Study the drawing (mm; zero at the part's minimum x, y, z) and answer. Give positions to 0.01 mm unless a question says otherwise; leave off trailing zeros. Order: outer loops, then holes, each group sorted by start corner. A loop starts at its lowest first (then second) coordinate and runs counter-clockwise, first axis right, second up. Notation, with made-up numbers: (-19, -25.75) - (16, -25.75) arc R29 ccw to (16, -0.75) - close; hole circle Ø10 at (71, 51.25). An arc over 180 degrees is marked (long way). Put each result on its own line as item: value.
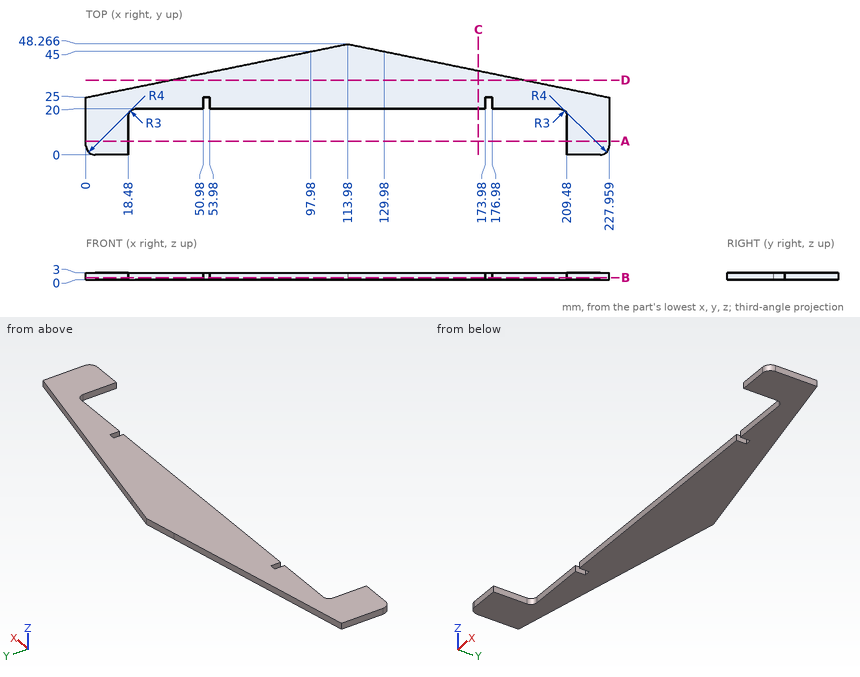
(1) Straight lines are drawn through the part: line 1 (X direction, y = 20.5, z = 1.2); line 2 (X direction, y = 13, z = 0.85); line 3 (Y direction, x = 138.5, z = 1). For each, find the intervals that lie inside material, in ascending order.
Geometry check:
line 1: x = 0 to 50.98, 53.98 to 173.98, 176.98 to 227.96
line 2: x = 0 to 18.48, 209.48 to 227.96
line 3: y = 20 to 43.26
(2) Section C-C, the plane x = 171 is taken. Write down the section's boundary in (y, z), then the cut area to 3 significant figures.
Geometry check:
outline: (20, 0) - (36.63, 0) - (36.63, 3) - (20, 3) - close
area: 49.9 mm²
(3) Section D-D, the plane y = 32.5 is taken. Write down the section's boundary in (x, z).
Geometry check:
outline: (36.74, 0) - (191.22, 0) - (191.22, 3) - (36.74, 3) - close
(4) Given pin 1 (1.5 mm diameter, centred on x = 117, z = 2, fed in from -Y); pin 2 (1.5 mm diameter, centred on x = 52, z = 1, fed in from -Y); pin 3 (3 mm diameter, centred on x = 182, y = 36.5, fed in from +Z), each flat-ended and moving along its own axis, determine where each tip first touches the part or whether it passes through.
Geometry check:
pin 1: stops at y = 20
pin 2: stops at y = 25
pin 3: passes through
(5) Section B-B, the plane z = 0.9 is taken. Write down the section's boundary in (x, y).
Geometry check:
outline: (0, 4) arc R4 ccw to (4, 0) - (18.48, 0) - (18.48, 17) arc R3 cw to (21.48, 20) - (50.98, 20) - (50.98, 25) - (53.98, 25) - (53.98, 20) - (173.98, 20) - (173.98, 25) - (176.98, 25) - (176.98, 20) - (206.48, 20) arc R3 cw to (209.48, 17) - (209.48, 0) - (223.96, 0) arc R4 ccw to (227.96, 4) - (227.96, 25) - (113.98, 48.27) - (0, 25) - close
(6) Section A-A, the plane y = 6 is taken. Write down the section's boundary in (x, z), then the cut area to 3 significant figures.
Geometry check:
outline: (0, 0) - (18.48, 0) - (18.48, 3) - (0, 3) - close; (209.48, 0) - (227.96, 0) - (227.96, 3) - (209.48, 3) - close
area: 111 mm²
